```python
from build123d import *

# Parameters (mm, degrees)
SKETCH_1_W          = 80
SKETCH_1_H          = 20
EXTRUDE_1_DEPTH     = 3
SKETCH_2_R          = 3.5
CUT_EXTRUDE_1_DEPTH = 3
SKETCH_3_W          = 15
SKETCH_3_H          = 4.5
CUT_EXTRUDE_2_DEPTH = 2
SKETCH_5_R          = 2.25
CUT_EXTRUDE_3_DEPTH = 2
SKETCH_6_W          = 4
SKETCH_6_H          = 20
EXTRUDE_2_DEPTH     = 15
CUT_EXTRUDE_4_DEPTH = 83
SKETCH_8_R          = 2
CUT_EXTRUDE_5_DEPTH = 83
SKETCH_9_W          = 4
SKETCH_9_H          = 20
EXTRUDE_3_DEPTH     = 25
SKETCH_10_R         = 3.5
CUT_EXTRUDE_6_DEPTH = 6
SKETCH_11_W         = 4.5
SKETCH_11_H         = 15
CUT_EXTRUDE_7_DEPTH = 3
SKETCH_12_R         = 2.25
CUT_EXTRUDE_8_DEPTH = 3
CUT_EXTRUDE_9_DEPTH = 10


with BuildPart() as part:
    # 草图1 → 凸台-拉伸1 (new body)
    with BuildSketch(Plane(origin=(0, 0, 0), x_dir=(1, 0, 0), z_dir=(0, 1, 0))):
        with Locations((40, -10)):
            Rectangle(SKETCH_1_W, SKETCH_1_H)
    extrude(amount=EXTRUDE_1_DEPTH)

    # 草图2 → 切除-拉伸1 (cut)
    with BuildSketch(Plane(origin=(0, 3, 0), x_dir=(1, 0, 0), z_dir=(0, 1, 0))):
        with Locations(Location((40, -10.045477327, 0), (0, 0, 270))):
            Circle(SKETCH_2_R)
    extrude(amount=-CUT_EXTRUDE_1_DEPTH, mode=Mode.SUBTRACT)

    # 草图3 → 切除-拉伸2 (cut)
    with BuildSketch(Plane(origin=(0, 3, 0), x_dir=(1, 0, 0), z_dir=(0, 1, 0))):
        with Locations((40, -10)):
            Rectangle(SKETCH_3_W, SKETCH_3_H)
    extrude(amount=-CUT_EXTRUDE_2_DEPTH, mode=Mode.SUBTRACT)

    # 草图5 → 切除-拉伸3 (cut)
    with BuildSketch(Plane(origin=(0, 3, 0), x_dir=(1, 0, 0), z_dir=(0, 1, 0))):
        with Locations((32.5, -10)):
            Circle(SKETCH_5_R)
        with Locations((47.5, -10)):
            Circle(SKETCH_5_R)
    extrude(amount=-CUT_EXTRUDE_3_DEPTH, mode=Mode.SUBTRACT)

    # 草图6 → 凸台-拉伸2 (add)
    with BuildSketch(Plane(origin=(0, 3, 0), x_dir=(1, 0, 0), z_dir=(0, 1, 0))):
        with Locations((2, -10)):
            Rectangle(SKETCH_6_W, SKETCH_6_H)
        with Locations((78, -10)):
            Rectangle(SKETCH_6_W, SKETCH_6_H)
        with Locations((59, -10)):
            Rectangle(SKETCH_6_W, SKETCH_6_H)
    extrude(amount=EXTRUDE_2_DEPTH)

    # 草图7 → 切除-拉伸4 (cut)
    with BuildSketch(Plane(origin=(80, 0, 0), x_dir=(0, 0, -1), z_dir=(1, 0, 0))):
        Polygon((-20, 13), (-15, 18), (-20, 18), align=None)
        Polygon((0, 13), (0, 18), (-5, 18), align=None)
    extrude(amount=-CUT_EXTRUDE_4_DEPTH, mode=Mode.SUBTRACT)

    # 草图8 → 切除-拉伸5 (cut)
    with BuildSketch(Plane.ZY):
        with Locations((5, 10.386894075)):
            Circle(SKETCH_8_R)
        with Locations((10, 10.386894075)):
            Circle(SKETCH_8_R)
        with Locations((15, 10.386894075)):
            Circle(SKETCH_8_R)
    extrude(amount=-CUT_EXTRUDE_5_DEPTH, mode=Mode.SUBTRACT)

    # 草图9 → 凸台-拉伸3 (add)
    with BuildSketch(Plane(origin=(0, 3, 0), x_dir=(1, 0, 0), z_dir=(0, 1, 0))):
        with Locations((21, -10)):
            Rectangle(SKETCH_9_W, SKETCH_9_H)
    extrude(amount=EXTRUDE_3_DEPTH)

    # 草图10 → 切除-拉伸6 (cut)
    with BuildSketch(Plane.ZY.offset(-19)):
        with Locations((10, 15.5)):
            Circle(SKETCH_10_R)
    extrude(amount=-CUT_EXTRUDE_6_DEPTH, mode=Mode.SUBTRACT)

    # 草图11 → 切除-拉伸7 (cut)
    with BuildSketch(Plane.ZY.offset(-19)):
        with Locations((10, 15.4)):
            Rectangle(SKETCH_11_W, SKETCH_11_H)
    extrude(amount=-CUT_EXTRUDE_7_DEPTH, mode=Mode.SUBTRACT)

    # 草图12 → 切除-拉伸8 (cut)
    with BuildSketch(Plane.ZY.offset(-19)):
        with Locations((10, 22.9)):
            Circle(SKETCH_12_R)
        with Locations((10, 7.9)):
            Circle(SKETCH_12_R)
    extrude(amount=-CUT_EXTRUDE_8_DEPTH, mode=Mode.SUBTRACT)

    # 草图13 → 切除-拉伸9 (cut)
    with BuildSketch(Plane.ZY.offset(-19)):
        Polygon((5, 28), (0, 23), (0, 28), align=None)
        Polygon((20, 28), (15, 28), (20, 23), align=None)
    extrude(amount=-CUT_EXTRUDE_9_DEPTH, mode=Mode.SUBTRACT)


solid = part.part
```
The listing builds one solid part. Answer for the finished solid, in the listing's coordinates (mm). A direction names the side the tool comes from. Coordinates: 2 decimals unless noted, no trailing zeros. Order: outer loops, then holes, each group sorted by start corner. A loop starts at its lowest first (then second) coordinate and runs counter-clockwise, first axis right, second up. Notation, with made-up numbers: M 0,61 L 54,61 A27 cw 54,84 Z; hole C -38.75,-11 d4. An arc over 180 degrees is marked long. Answer as a JSON object with one key per item and string values. Group by question number.
1. Section B-B on y = 13.75 is taken. Write down the section's boundary in (x, z).
2. Determine the mould class of faces 5 (the cylindrical face through (77.972, 9.17, 8.413)), 6 (the flat face through (68, 3, 10)), 7 (the flat face through (2, 15, 18)) for opening direction Z: released by +Z, released by -Z, zero draft, split by the parting line, or undercut.
3. Section A-A on x = 40 is taken. Write down the section's boundary in (y, z).
4. Section D-D on x = 29.5 is taken. Write down the section's boundary in (y, z), then the cut area to 3 significant figures.
5. Flat-ended cylindrical pins translate along their axes: P1, Ø1.5, axis at x = 28, z = 10.5, coming from the +Y side; P2, Ø4.5, axis at y = 10.39, z = 15, coming from the +X side; P3, Ø3.5, axis at y = 10.39, z = 15, coming from the -X side; P4, Ø3, axis at y = 10.39, z = 5, coming from the +X side. Find the tip coordinate at first contact, or state that the pin passes through.
6. A tool of negligible diameter and unlimited length cuts with its end or side. For faces 1 (the cylindrical face through (1.972, 9.17, 13.413)), 2 (the flat face through (59, 18, 10)), 3 (the cylindrical face through (21.416, 15.654, 6.503)), 4 (the flat face through (4, 10.4, 12.4)), from which of +Z, -Z, +X, -X, +Y, -Y can it reach the whole face along a straight path? Write none if from no direction.
7. Section C-C on z = 2 is taken. Write down the section's boundary in (x, y), then the cut area to 3 significant figures.
8. Straight lines are drawn through the part: line 1 (X direction, y = 5.5, z = 11.75); line 2 (X direction, y = 13, z = 11.25); line 3 (Z direction, x = 20.4, y = 15.5). For each, find the intervals that lie inside material, in ascending order.
Values follow:
{
 "1": {"outline": "M 0,0.75 L 4,0.75 L 4,19.25 L 0,19.25 Z; M 19,0 L 23,0 L 23,6.97 L 19,6.97 Z; M 19,13.03 L 23,13.03 L 23,20 L 19,20 Z; M 57,0.75 L 61,0.75 L 61,19.25 L 57,19.25 Z; M 76,0.75 L 80,0.75 L 80,19.25 L 76,19.25 Z"},
 "2": {"face 5": "undercut", "face 6": "zero draft", "face 7": "released by +Z"},
 "3": {"outline": "M 0,0 L 3,0 L 3,6.55 L 0,6.55 Z; M 0,13.55 L 3,13.55 L 3,20 L 0,20 Z"},
 "4": {"outline": "M 0,0 L 3,0 L 3,20 L 0,20 Z", "area": "60.0 mm2"},
 "5": {"P1": "y = 3", "P2": "x = 80", "P3": "x = 19", "P4": "x = 23"},
 "6": {"face 1": "-X", "face 2": "+Z, -Z, +X, +Y", "face 3": "none", "face 4": "+Z, -Z, +Y"},
 "7": {"outline": "M 0,0 L 80,0 L 80,15 L 76,15 L 76,3 L 61,3 L 61,15 L 57,15 L 57,3 L 23,3 L 23,25 L 19,25 L 19,3 L 4,3 L 4,15 L 0,15 Z", "area": "472 mm2"},
 "8": {"line 1": "0 to 4, 19 to 23, 57 to 61, 76 to 80", "line 2": "0 to 4, 57 to 61, 76 to 80", "line 3": "0 to 6.5, 13.5 to 20"}
}
